Part model, mm, in its own coordinate system. Round coordinates to 2 decimals unless told otherwise and drop trailing zeros. Order: outer loops, then holes, each group sorted by start corner. A loop starts at its lowest first (then second) coordinate and runs counter-clockwise, first axis right, second up. Notation, with made-up numbers: (-6, 12) - (46, 12) arc R20 ccw to (46, 48) - close; hole circle Ø11 at (88.5, -15.5). An arc over 180 degrees is marked (long way). Answer as a JSON object with one key per item and string values.
```python
from build123d import *

# Parameters (mm, degrees)
SKETCH_R     = 49
PAD_DEPTH    = 2
SKETCH001_R  = 45.5
PAD001_DEPTH = 6.35
SKETCH002_R  = 15
POCKET_DEPTH = 6.351
CHAMFER_SIZE = 0.6


with BuildPart() as part:
    # Sketch → Pad (new body)
    with BuildSketch(Plane.XY):
        Circle(SKETCH_R)
    extrude(amount=PAD_DEPTH)

    # Sketch001 → Pad001 (join)
    with BuildSketch(Plane.XY):
        Circle(SKETCH001_R)
    extrude(amount=PAD001_DEPTH)

    # Sketch002 → Pocket (cut, through all)
    with BuildSketch(Plane.XY):
        Circle(SKETCH002_R)
    extrude(amount=POCKET_DEPTH, mode=Mode.SUBTRACT)

    # Chamfer
    chamfer_edges = [part.edges().sort_by_distance(p)[0] for p in [
        (-45.5, 0, 6.35),
        (-15, 0, 6.35),
        (-49, 0, 0),
        (-15, 0, 0),
    ]]
    chamfer(chamfer_edges, length=CHAMFER_SIZE)


solid = part.part
```
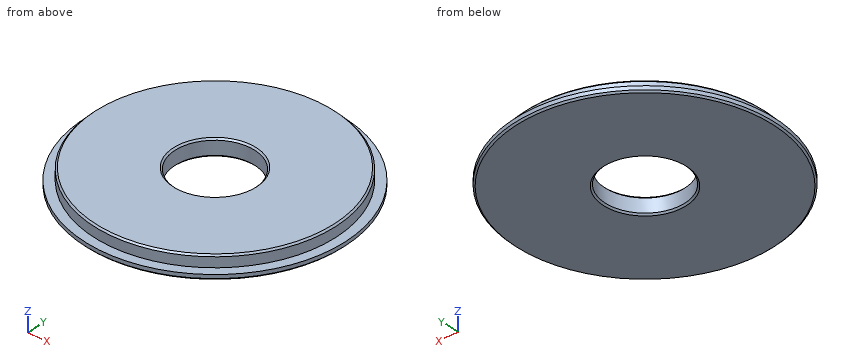
Item 1: Cut at A-A (y = 0). Write the cut outline in (x, z), plus the area to 3 significant figures.
Taken from the geometry:
{"outline": "(-49, 0.6) - (-48.4, 0) - (-15.6, 0) - (-15, 0.6) - (-15, 5.75) - (-15.6, 6.35) - (-44.9, 6.35) - (-45.5, 5.75) - (-45.5, 2) - (-49, 2) - close; (15, 0.6) - (15.6, 0) - (48.4, 0) - (49, 0.6) - (49, 2) - (45.5, 2) - (45.5, 5.75) - (44.9, 6.35) - (15.6, 6.35) - (15, 5.75) - close", "area": "400 mm2"}
Item 2: Cut at C-C (z = 3.25). Write the cut outline in (x, y).
Taken from the geometry:
{"outline": "circle Ø91 at (0, 0); hole circle Ø30 at (0, 0)"}
Item 3: Drop flat-ended pins along their axis: P1, Ø2, axis at x = 36, y = 26, coming from the -Z side; P2, Ø3, axis at x = 13.5, z = 3, coming from the +Y side; P3, Ø2, axis at y = -2.5, z = 2.5, coming from the +X side; P4, Ø18, axis at x = 0, y = 0, coming from the +Z side (1 decimal). Give the stop position or say it passes through.
Taken from the geometry:
{"P1": "z = 0", "P2": "y = 47.41", "P3": "x = 48.97", "P4": "through"}
Item 4: Probe L1, parallel to X at y = 0, z = 4.65; L2, parallel to X at y = -8, z = 3. List the from-to ranges inside material, lowest first. Write a range as from..to.
Taken from the geometry:
{"L1": "-45.5..-15, 15..45.5", "L2": "-44.79..-12.69, 12.69..44.79"}
